Here's the drawing with two shaded views (mm, measured from the low corner). I have some questions. Give positions to 0.01 mm unless a question says otherwise; leave off trailing zeros. Write each loop counter-clockwise with the first axis right and the second up, starting at its lowest first coordinate (ties: lowest second). Pieces come first, ordered by that corner, then holes. Notation, with made-up numbers: (88.25, 36.25) -> (136.25, 36.25) arc R11 cw to (136.25, 45.25) -> close; hole circle Ø7 at (23.25, 67.5). An arc over 180 degrees is marked (long way). One line per question, with ' | ' between items.
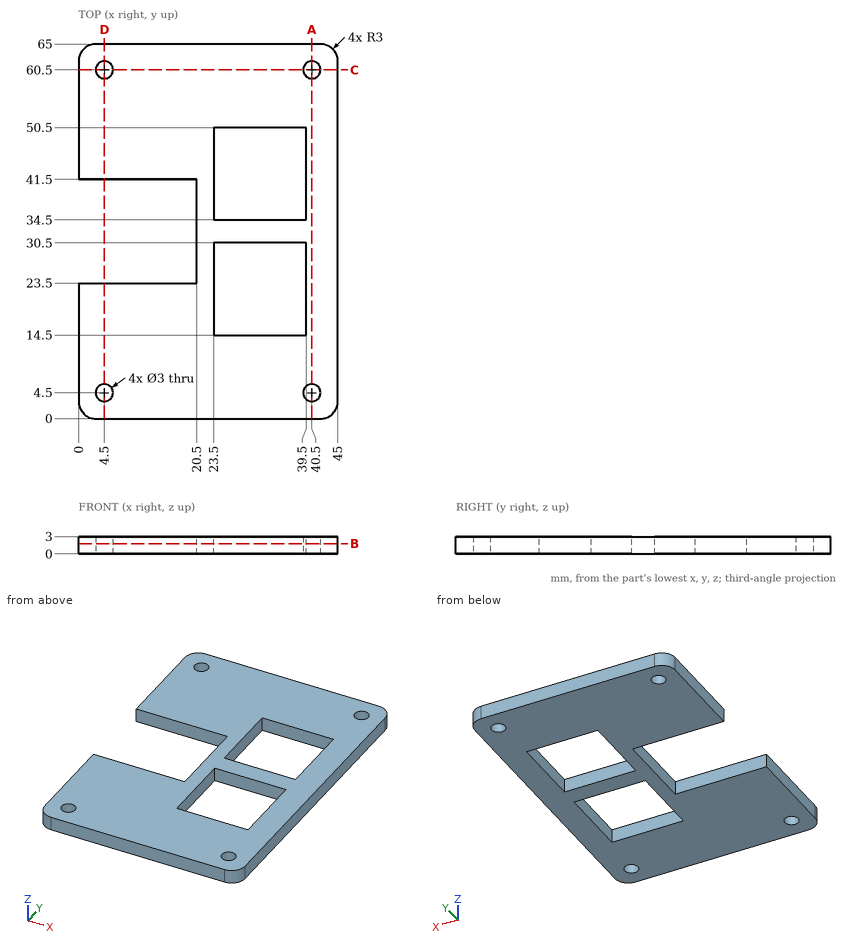
Q1. Will these pins go through, and if not, where does the flat tip stop? pin 1 (0.9 mm diameter, centred on x = 32, z = 2, fed in from -Y); pin 2 (1.5 mm diameter, centred on y = 40.5, z = 1.5, fed in from -X).
Answer below:
pin 1: stops at y = 0 | pin 2: stops at x = 20.5
Q2. Imagine slicing it at D-D on x = 4.5. Please give me the cut outline in (y, z).
Answer below:
outline: (0, 0) -> (3, 0) -> (3, 3) -> (0, 3) -> close; (6, 0) -> (23.5, 0) -> (23.5, 3) -> (6, 3) -> close; (41.5, 0) -> (59, 0) -> (59, 3) -> (41.5, 3) -> close; (62, 0) -> (65, 0) -> (65, 3) -> (62, 3) -> close
Q3. Imagine slicing it at C-C on y = 60.5. Please give me the cut outline in (x, z).
Answer below:
outline: (0, 0) -> (3, 0) -> (3, 3) -> (0, 3) -> close; (6, 0) -> (39, 0) -> (39, 3) -> (6, 3) -> close; (42, 0) -> (45, 0) -> (45, 3) -> (42, 3) -> close
Q4. Imagine slicing it at A-A on x = 40.5. Please give me the cut outline in (y, z).
Answer below:
outline: (0, 0) -> (3, 0) -> (3, 3) -> (0, 3) -> close; (6, 0) -> (59, 0) -> (59, 3) -> (6, 3) -> close; (62, 0) -> (65, 0) -> (65, 3) -> (62, 3) -> close
Q5. If I drill on line 1 along Y through (x, z) = (33, 0.3); line 2 along Y through (x, z) = (4.5, 1.3); line 3 along Y through (x, z) = (40.5, 1.9), over which ranges is the centre line in solid material (lowest first)?
Answer below:
line 1: y = 0 to 14.5, 30.5 to 34.5, 50.5 to 65 | line 2: y = 0 to 3, 6 to 23.5, 41.5 to 59, 62 to 65 | line 3: y = 0 to 3, 6 to 59, 62 to 65
Q6. Imagine slicing it at B-B on z = 1.8. Please give me the cut outline in (x, y), and give its area (3 significant figures).
Answer below:
outline: (0, 3) arc R3 ccw to (3, 0) -> (42, 0) arc R3 ccw to (45, 3) -> (45, 62) arc R3 ccw to (42, 65) -> (3, 65) arc R3 ccw to (0, 62) -> (0, 41.5) -> (20.5, 41.5) -> (20.5, 23.5) -> (0, 23.5) -> close; hole circle Ø3 at (4.5, 4.5); hole circle Ø3 at (4.5, 60.5); hole (23.5, 14.5) -> (39.5, 14.5) -> (39.5, 30.5) -> (23.5, 30.5) -> close; hole (23.5, 34.5) -> (39.5, 34.5) -> (39.5, 50.5) -> (23.5, 50.5) -> close; hole circle Ø3 at (40.5, 4.5); hole circle Ø3 at (40.5, 60.5) | area: 2,010 mm^2
